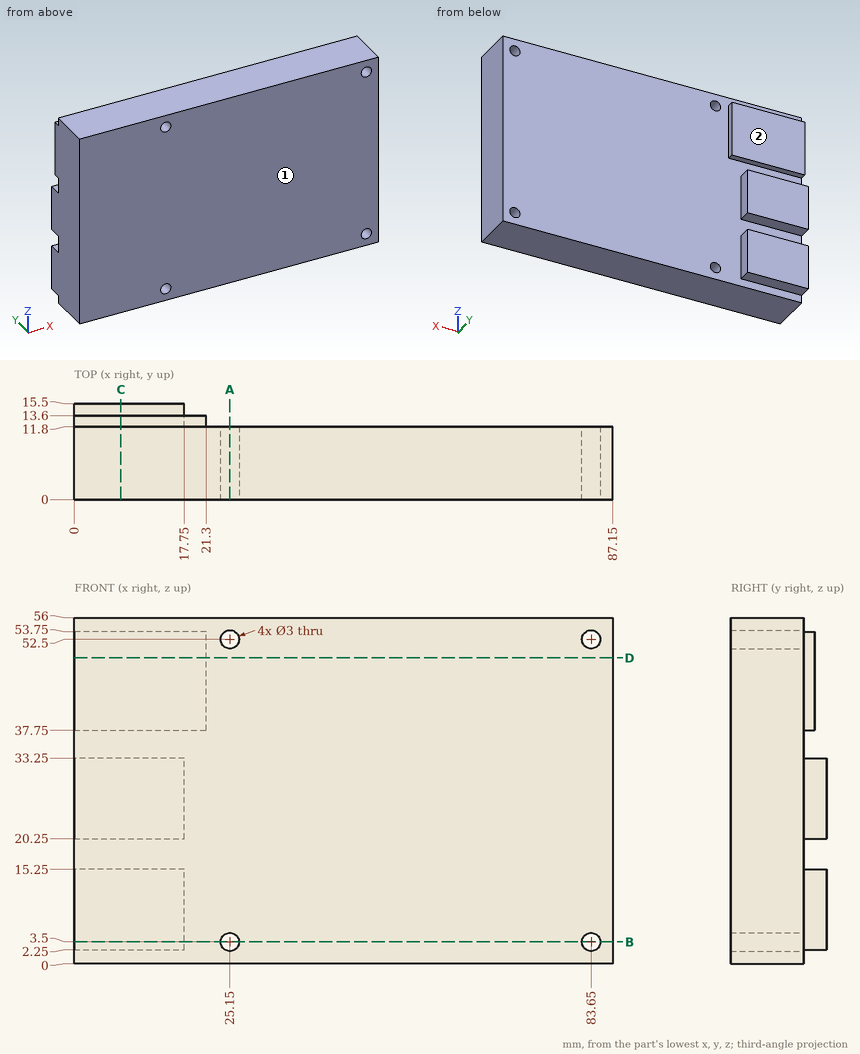
Drawing for the job (mm, zero at the part's lowest x, y, z). A direction names the side the tool comes from. Coordinates: 2 decimals unless noted, no trailing zeros. Order: outer loops, then holes, each group sorted by start corner. A loop starts at its lowest first (then second) coordinate and runs counter-clockwise, first axis right, second up. Notation, with made-up numbers: (-19, 72.5) -> (7, 72.5) arc R32 ccw to (7, 106.5) -> close; hole circle Ø7 at (24.5, 77). An arc over 180 degrees is marked (long way). Answer in a Markdown table with one row per item.
1) Band-saw the part on D-D (z = 49.5). List the corners of the cut face in (x, y), and give its area (3 significant figures).
Check values:
| item | result |
|---|---|
| outline | (0, 0) -> (87.15, 0) -> (87.15, 11.8) -> (21.3, 11.8) -> (21.3, 13.6) -> (0, 13.6) -> close |
| area | 1,070 mm2 |
2) Band-saw the part on A-A (x = 25.15). List the corners of the cut face in (y, z), and give its area (3 significant figures).
Check values:
| item | result |
|---|---|
| outline | (0, 0) -> (11.8, 0) -> (11.8, 2) -> (0, 2) -> close; (0, 5) -> (11.8, 5) -> (11.8, 51) -> (0, 51) -> close; (0, 54) -> (11.8, 54) -> (11.8, 56) -> (0, 56) -> close |
| area | 590 mm2 |
3) Which spindle directions (+Z, -Z, +X, -X, +Y, -Y) get a long thin tool onto all of the face, cutting with end or side? Do the marked faces 1 and 2. Say none if no direction does.
Check values:
| item | result |
|---|---|
| face 1 | +Z, -Z, +X, -X, -Y |
| face 2 | +Z, +X, -X, +Y |
4) Drill centre lines: line 1 (X direction, y = 3, z = 3.5); line 2 (Z direction, x = 83.65, y = 4); line 3 (Z direction, x = 10, y = 14.25). Where is each one in solid material? Low to high.
Check values:
| item | result |
|---|---|
| line 1 | 0 to 23.65, 26.65 to 82.15, 85.15 to 87.15 |
| line 2 | 0 to 2, 5 to 51, 54 to 56 |
| line 3 | 2.25 to 15.25, 20.25 to 33.25 |
5) Flat gauge pins, fed straight in: P1, Ø4, axis at y = 14.5, z = 9, coming from the +X side; P2, Ø3, axis at x = 5, y = 14, coming from the -Z side; P3, Ø17, axis at x = 53.5, z = 37.5, coming from the +Y side. Where does each tip first touch, or does it go through?
Check values:
| item | result |
|---|---|
| P1 | x = 17.75 |
| P2 | z = 2.25 |
| P3 | y = 11.8 |
6) Band-saw the part on C-C (x = 7.5). List the corners of the cut face in (y, z), and give its area (3 significant figures).
Check values:
| item | result |
|---|---|
| outline | (0, 0) -> (11.8, 0) -> (11.8, 2.25) -> (15.5, 2.25) -> (15.5, 15.25) -> (11.8, 15.25) -> (11.8, 20.25) -> (15.5, 20.25) -> (15.5, 33.25) -> (11.8, 33.25) -> (11.8, 37.75) -> (13.6, 37.75) -> (13.6, 53.75) -> (11.8, 53.75) -> (11.8, 56) -> (0, 56) -> close |
| area | 786 mm2 |
7) Band-saw the part on B-B (z = 3.5). List the corners of the cut face in (x, y), and give its area (3 significant figures).
Check values:
| item | result |
|---|---|
| outline | (0, 0) -> (23.65, 0) -> (23.65, 11.8) -> (17.75, 11.8) -> (17.75, 15.5) -> (0, 15.5) -> close; (26.65, 0) -> (82.15, 0) -> (82.15, 11.8) -> (26.65, 11.8) -> close; (85.15, 0) -> (87.15, 0) -> (87.15, 11.8) -> (85.15, 11.8) -> close |
| area | 1,020 mm2 |
